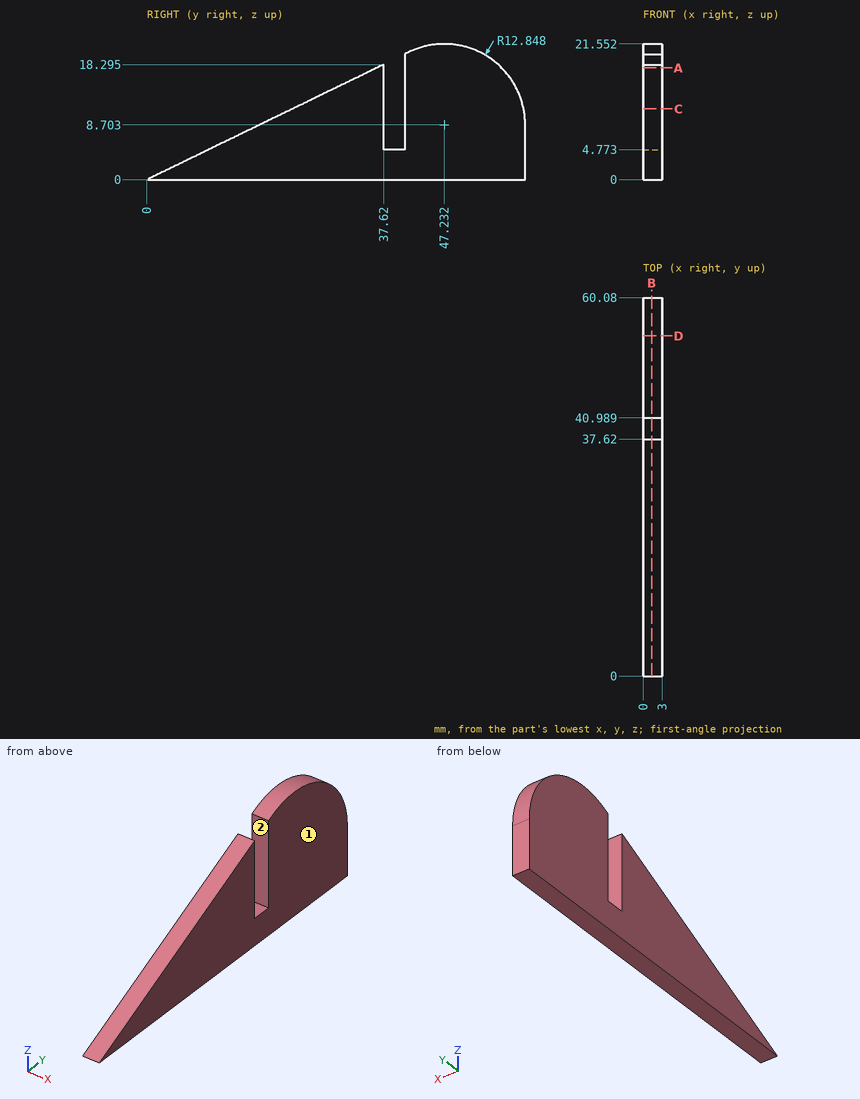
Check sheet for the drawn part. Datum: minimum x, y, z corner. Units: mm. A direction names the side the tool comes from. Round coordinates to 2 decimals unless told otherwise and drop trailing zeros. Order: outer loops, then holes, each group sorted by start corner. A loop starts at its lowest first (then second) coordinate and runs counter-clockwise, first axis right, second up.
1. Access from +Z, -Z, +X, -X, +Y, -Y to the whole of each face (thin tool, end or side, straight path). Record for the marked faces 1 and 2.
Final values:
face 1: +Z, -Z, +X, +Y, -Y
face 2: +Z, +X, -X
2. Section check A-A on z = 17.75. Record the cut outline in (x, y) (1 decimal).
Final values:
outline: (0, 36.5) - (3, 36.5) - (3, 37.6) - (0, 37.6) - close; (0, 41) - (3, 41) - (3, 56.4) - (0, 56.4) - close
3. Section check C-C on z = 11.25. Record the cut outline in (x, y) (1 decimal).
Final values:
outline: (0, 23.1) - (3, 23.1) - (3, 37.6) - (0, 37.6) - close; (0, 41) - (3, 41) - (3, 59.8) - (0, 59.8) - close
4. Section check B-B on x = 1.35. Record the cut outline in (y, z) (1 decimal), then the cut area to 3 significant figures.
Final values:
outline: (0, 0) - (60.1, 0) - (60.1, 8.7) arc R12.8 ccw to (41, 19.9) - (41, 4.8) - (37.6, 4.8) - (37.6, 18.3) - close
area: 733 mm2
5. Thickness scan on L1, parallel to Z at x = 1.05, y = 39.5; L2, parallel to Y at x = 0.8, z = 9.5 (1 decimal); L3, parallel to Y at x = 1.9, z = 6.5 (1 decimal). Record the ranges inside material, lowest first.
Final values:
L1: z = 0 to 4.77
L2: y = 19.5 to 37.6, 41 to 60.1
L3: y = 13.4 to 37.6, 41 to 60.1
6. Go/stop test with flat-tipped pins: P1, Ø1.5, axis at x = 1, z = 14, coming from the -Y side (1 decimal); P2, Ø1.5, axis at x = 1, y = 11.5, coming from the +Z side; P3, Ø1.5, axis at x = 1.5, z = 8, coming from the -Y side. Record where each tip stops, or that it passes through.
Final values:
P1: stops at y = 27.2
P2: stops at z = 5.96
P3: stops at y = 14.91
7. Section check D-D on y = 54. Record the cut outline in (x, z) (1 decimal).
Final values:
outline: (0, 0) - (3, 0) - (3, 19.6) - (0, 19.6) - close
